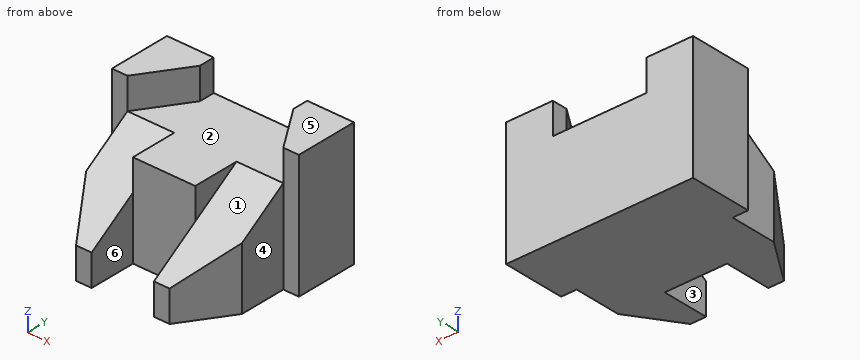
from build123d import *

# Parameters (mm, degrees)
BOSS_EXTRUDE1_DEPTH = 60
BOSS_EXTRUDE2_DEPTH = 20
CUT_EXTRUDE1_DEPTH  = 30
CUT_EXTRUDE2_DEPTH  = 30


with BuildPart() as part:
    # Sketch1 → Boss-Extrude1 (new body)
    with BuildSketch(Plane.XY):
        Polygon((0, 0), (10, 0), (10, 30), (50, 30), (50, 0), (60, 0), (80, 30), (80, 60), (90, 60), (90, 100), (-30, 100), (-30, 60), (-20, 60), (-20, 30), align=None)
    extrude(amount=BOSS_EXTRUDE1_DEPTH)

    # Sketch2 → Boss-Extrude2 (add)
    with BuildSketch(Plane.XY.offset(60)):
        Polygon((-20, 60), (0, 90), (0, 100), (-30, 100), (-30, 60), align=None)
        Polygon((80, 60), (60, 90), (60, 100), (90, 100), (90, 60), align=None)
    extrude(amount=BOSS_EXTRUDE2_DEPTH)

    # Sketch3 → Cut-Extrude1 (cut)
    with BuildSketch(Plane.ZY.offset(20)):
        Polygon((60, 60), (20, 0), (60, 0), align=None)
    extrude(amount=-CUT_EXTRUDE1_DEPTH, mode=Mode.SUBTRACT)

    # Sketch4 → Cut-Extrude2 (cut)
    with BuildSketch(Plane(origin=(80, 0, 0), x_dir=(0, 0, -1), z_dir=(1, 0, 0))):
        Polygon((-60, 60), (-20, 0), (-60, 0), align=None)
    extrude(amount=-CUT_EXTRUDE2_DEPTH, mode=Mode.SUBTRACT)


solid = part.part
Input: part model. Units: mm. Frame: model coordinates. Face numbers are marked on the shaded views. A direction names the side the tool comes from. Give positions to 0.01 mm unless a question says otherwise; leave off trailing zeros. Loops run counter-clockwise (first coordinate to the right, second up) from the corner with the lowest first, then second, coordinate; pieces in that order, holes last. Notation, with made-up numbers: (53.25, 36.25) - (96.25, 36.25) arc R21 ccw to (96.25, 67.25) - close; hole circle Ø6 at (-22, -40). An arc over 180 degrees is marked (long way). Use CSV: the item, a comma, the result in double quotes. Start each with the question number.
Item 1: Section B-B on y = 21. Return loops of the section in (x, z), then the cut area to 3 significant figures.
Item 2: Section A-A on z = 32. Return loops of the section in (x, y), then the cut area to 3 significant figures.
Item 3: Section D-D on y = 58.5. Return loops of the section in (x, z), then the cut area to 3 significant figures.
Item 4: Line query: line 1 (Y direction, x = 34, z = 20); line 2 (X direction, y = 89.5, z = 65); line 3 (Y direction, x = 82, z = 6.5). Output: solid intervals per line, ascending.
Item 5: Reachability of the marked faces 1, 2 and 3 from +Z, -Z, +X, -X, +Y, -Y: full face, straight path, thin tool, end or side. Return the list, or none.
Item 6: Contact query for flat-ended pins moving along their axis: P1, Ø15, axis at y = 8, z = 19.5, coming from the +X side; P2, Ø11, axis at x = 86.5, z = 48.5, coming from the -Y side; P3, Ø12, axis at x = 35.5, z = 17.5, coming from the -Y side. Output: stop coordinate, or through.
Item 7: Section C-C on x = 64. Return loops of the section in (y, z).
Item 8: Mould query, pull axis X, two halves, no side actions, for the marked faces 4, 5 and 6. Classes: pulls with the +X half, pulls with the -X half, needs draft (parallel to the pull), parting line crosses it, or undercut.
Ans:
1,outline,"(-14, 0) - (10, 0) - (10, 34) - (-14, 34) - close; (50, 0) - (74, 0) - (74, 34) - (50, 34) - close"
1,area,"1,630 mm2"
2,outline,"(-30, 60) - (-20, 60) - (-20, 30) - (-12, 18) - (10, 18) - (10, 30) - (50, 30) - (50, 18) - (72, 18) - (80, 30) - (80, 60) - (90, 60) - (90, 100) - (-30, 100) - close"
2,area,"8,420 mm2"
3,outline,"(-20, 0) - (80, 0) - (80, 59) - (50, 59) - (50, 60) - (10, 60) - (10, 59) - (-20, 59) - close"
3,area,"5,940 mm2"
4,line 1,"y = 30 to 100"
4,line 2,"x = -30 to -0.33, 60.33 to 90"
4,line 3,"y = 60 to 100"
5,face 1,"+Z, +X, -Y"
5,face 2,"+Z, -Y"
5,face 3,"+Z, -Z, -Y"
6,P1,"stops at x = 70.33"
6,P2,"stops at y = 60"
6,P3,"stops at y = 30"
7,outline,"(6, 0) - (100, 0) - (100, 80) - (84, 80) - (84, 60) - (60, 60) - (6, 24) - close"
8,face 4,"pulls with the +X half"
8,face 5,"needs draft"
8,face 6,"undercut"
